Design review of the part shown in the three views and the two pictorial views. Dimensions are in mm from the part's minimum x, y and z. A direction names the side the tool comes from. Give positions to 0.01 mm unless a question says otherwise; leave off trailing zeros. Loops run counter-clockwise (first coordinate to the right, second up) from the corner with the lowest first, then second, coordinate; pieces in that order, holes last. Notation, with made-up numbers: (86, 44) - (126, 44) arc R15 ccw to (126, 66) - close; hole circle Ø4 at (-24, 68.25). An arc over 180 degrees is marked (long way). Answer in a Markdown table with one row per item.
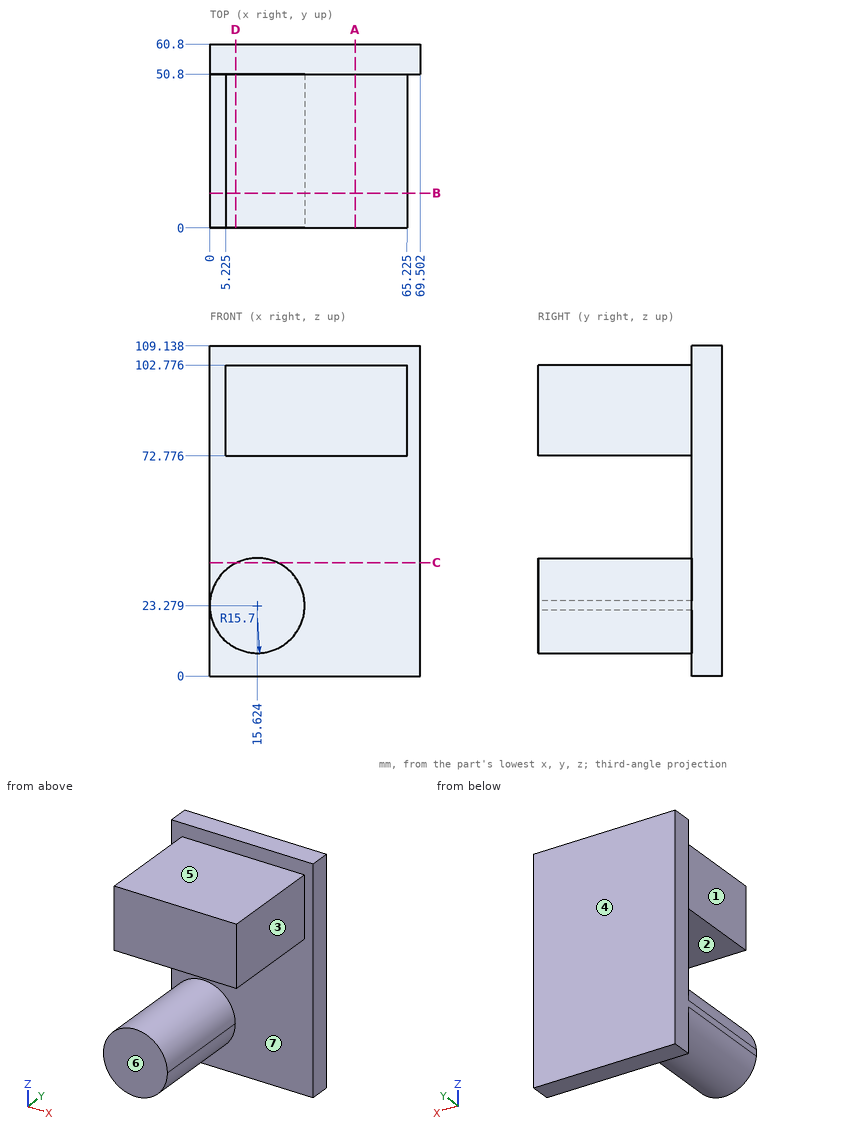
1. Clearance check with flat-ended pins moving along their axes: pin 1 (10 mm diameter, centred on y = 42, z = 78.5, fed in from -X) (1 decimal); pin 2 (8 mm diameter, centred on y = 34, z = 40.5, fed in from -X) (1 decimal); pin 3 (10 mm diameter, centred on y = 29.5, z = 36.5, fed in from -X); pin 4 (4 mm diameter, centred on x = 36.5, z = 94, fed in from -Y). State where each tip first meets the part, or that it passes through.
Values:
| item | result |
|---|---|
| pin 1 | stops at x = 5.2 |
| pin 2 | stops at x = 7.2 |
| pin 3 | stops at x = 2.25 |
| pin 4 | stops at y = 0 |
2. For the marked faces 1, 2, 3 and 4, list the 3-axis set-ups (+Z, -Z, +X, -X, +Y, -Y) from which the entire face can be reached by the end or side of a thin tool; tool diameter is ignored.
Values:
| item | result |
|---|---|
| face 1 | +Z, -X, -Y |
| face 2 | +X, -X, -Y |
| face 3 | +Z, -Z, +X, -Y |
| face 4 | +Z, -Z, +X, -X, +Y |
3. We need section D-D, the plane x = 8.5. Give the boundary of the cut face in (y, z) (1 decimal).
Values:
| item | result |
|---|---|
| outline | (0, 9.3) - (50.8, 9.3) - (50.8, 0) - (60.8, 0) - (60.8, 109.1) - (50.8, 109.1) - (50.8, 102.8) - (0, 102.8) - (0, 72.8) - (50.8, 72.8) - (50.8, 37.3) - (0, 37.3) - close |
4. Wall thickness on line 1 (Z direction, x = 38, y = 40) (1 decimal); line 2 (Y direction, x = 49.5, z = 20); line 3 (Z direction, x = 29, y = 10) (1 decimal): over which ranges is each line inside the solid? List them lowest first. Write a range as [from, to].
Values:
| item | result |
|---|---|
| line 1 | z = [72.8, 102.8] |
| line 2 | y = [50.8, 60.8] |
| line 3 | z = [15.1, 31.5], [72.8, 102.8] |
5. Mouldability with a two-part tool opening along Z and no side actions: class the marked faces 5, 6 and 7 as released by +Z, released by -Z, zero draft, split by the parting line, or undercut.
Values:
| item | result |
|---|---|
| face 5 | released by +Z |
| face 6 | zero draft |
| face 7 | undercut |
6. We need section B-B, the plane y = 11.5. Give the boundary of the cut face in (x, z) (1 decimal), and give its area (3 significant figures).
Values:
| item | result |
|---|---|
| outline | (0, 21.7) arc R15.7 ccw (long way) to (0, 24.8) - close; (5.2, 72.8) - (65.2, 72.8) - (65.2, 102.8) - (5.2, 102.8) - close |
| area | 2,570 mm^2 |
7. We need section C-C, the plane z = 37.5. Give the boundary of the cut face in (x, y).
Values:
| item | result |
|---|---|
| outline | (0, 50.8) - (8.97, 50.8) - (8.97, 0) - (22.28, 0) - (22.28, 50.8) - (69.5, 50.8) - (69.5, 60.8) - (0, 60.8) - close |
8. We need section A-A, the plane x = 48. Give the boundary of the cut face in (y, z) (1 decimal), and give its area (3 significant figures).
Values:
| item | result |
|---|---|
| outline | (0, 72.8) - (50.8, 72.8) - (50.8, 0) - (60.8, 0) - (60.8, 109.1) - (50.8, 109.1) - (50.8, 102.8) - (0, 102.8) - close |
| area | 2,620 mm^2 |
